```python
from build123d import *

# Parameters (mm, degrees)
F0_W     = 76
F0_H     = 54
F0_H_2   = 18
F1_DEPTH = 64
F2_T     = -13
F3_R     = 12.5
F4_DEPTH = 103.3


with BuildPart() as f1:
    # F0 (on Front) → F1 (new body)
    with BuildSketch(Plane.XZ):
        with Locations((1.435856, 13.840802)):
            Rectangle(F0_W, F0_H)
        with Locations((1.435856, -22.159198)):
            Rectangle(F0_W, F0_H_2)
    extrude(amount=-F1_DEPTH)

    # F2
    f2_openings = [f1.faces().sort_by_distance(p)[0] for p in [
        (1.435856, 32, 40.840802),
    ]]
    offset(amount=F2_T, openings=f2_openings)

    # F3 (on face) → F4 (cut)
    with BuildSketch(Plane.YZ.offset(39.435856)):
        with Locations((32, 4.840802)):
            Circle(F3_R)
    extrude(amount=-F4_DEPTH, mode=Mode.SUBTRACT)


solid = f1.part
```
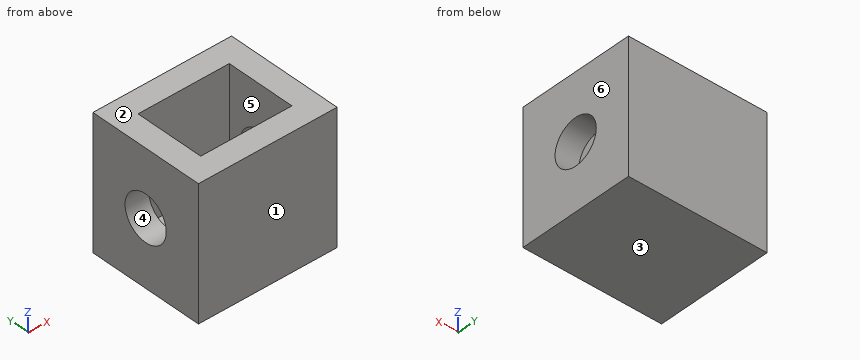
For this review, take the finished solid that the model builds, in its own axes (mm). Face numbers are marked on the shaded views. A direction names the side the tool comes from. Coordinates: 2 decimals unless noted, no trailing zeros. Loops run counter-clockwise (first coordinate to the right, second up) from the corner with the lowest first, then second, coordinate; pieces in that order, holes last. Notation, with made-up numbers: (80, -9.5) -> (121, -9.5) arc R31 cw to (121, 18.5) -> close; hole circle Ø1 at (36.5, 14.25). An arc over 180 degrees is marked (long way). Return JSON: item names as keys, results as strings. Group by question number.
(1) Consider section C-C, the plane z = -1.5. Give the boundary of the cut face in (x, y), plus the area to 3 significant figures.
(2) For pin 1 Ø20 at (y, z) = (32, 4.84) entering from -X; pin 2 Ø19 at (x, y) = (0.5, 30) entering from +Z, all flat-tipped, find the tip position at first contact; note any pin that passes through.
(3) To check wall thickness, follow L1, parallel to Y at x = 17, z = 21.5; L2, parallel to X at y = 14, z = 0; L3, parallel to Z at x = 29, y = 32. State the ranges of each line that lie inside material, in increasing order.
(4) Tool access review of the marked faces 5 and 6: name each direction out of +Z, -Z, +X, -X, +Y, -Y from which nothing blocks a thin tool from reaching the whole face with its end or side.
(5) Mouldability with a two-part tool opening along Z and no side actions: class the marked faces 1, 2, 3 and 4 as pulls with the +Z half, pulls with the -Z half, needs draft (parallel to the pull), parting line crosses it, or undercut.
(6) Consider section A-A, the plane y = 32. Give the boundary of the cut face in (x, z), plus the area to 3 significant figures.
(7) Consider section B-B, the plane z = 33. Give the boundary of the cut face in (x, y).
(8) Consider section D-D, the plane x = 13. Give the boundary of the cut face in (y, z), plus the area to 3 significant figures.
Results below:
{
 "1": {"outline": "(-36.56, 0) -> (39.44, 0) -> (39.44, 21.23) -> (26.44, 21.23) -> (26.44, 13) -> (-23.56, 13) -> (-23.56, 21.23) -> (-36.56, 21.23) -> close; (-36.56, 42.77) -> (-23.56, 42.77) -> (-23.56, 51) -> (26.44, 51) -> (26.44, 42.77) -> (39.44, 42.77) -> (39.44, 64) -> (-36.56, 64) -> close", "area": "2,400 mm2"},
 "2": {"pin 1": "passes through", "pin 2": "stops at z = -18.16"},
 "3": {"L1": "y = 0 to 13, 51 to 64", "L2": "x = -36.56 to -23.56, 26.44 to 39.44", "L3": "z = -31.16 to -7.66, 17.34 to 40.84"},
 "4": {"face 5": "+Z", "face 6": "+Z, -Z, +X, +Y, -Y"},
 "5": {"face 1": "needs draft", "face 2": "pulls with the +Z half", "face 3": "pulls with the -Z half", "face 4": "undercut"},
 "6": {"outline": "(-36.56, -31.16) -> (39.44, -31.16) -> (39.44, -7.66) -> (26.44, -7.66) -> (26.44, -18.16) -> (-23.56, -18.16) -> (-23.56, -7.66) -> (-36.56, -7.66) -> close; (-36.56, 17.34) -> (-23.56, 17.34) -> (-23.56, 40.84) -> (-36.56, 40.84) -> close; (26.44, 17.34) -> (39.44, 17.34) -> (39.44, 40.84) -> (26.44, 40.84) -> close", "area": "1,870 mm2"},
 "7": {"outline": "(-36.56, 0) -> (39.44, 0) -> (39.44, 64) -> (-36.56, 64) -> close; hole (-23.56, 13) -> (26.44, 13) -> (26.44, 51) -> (-23.56, 51) -> close"},
 "8": {"outline": "(0, -31.16) -> (64, -31.16) -> (64, 40.84) -> (51, 40.84) -> (51, -18.16) -> (13, -18.16) -> (13, 40.84) -> (0, 40.84) -> close", "area": "2,370 mm2"}
}
